```python
from build123d import *

# Parameters (mm, degrees)
SKETCH1_W           = 151.13
SKETCH1_H           = 82.55
BOSS_EXTRUDE1_DEPTH = 15.875
SKETCH2_W           = 167.005
SKETCH2_H           = 98.425
BOSS_EXTRUDE2_DEPTH = 3.81
FILLET2_R           = 6.35
CUT_EXTRUDE1_DEPTH  = 184.691243225
CUT_EXTRUDE3_DEPTH  = 5.4356
SKETCH5_W           = 8.89
SKETCH5_H           = 6.35
CUT_EXTRUDE4_DEPTH  = 189.417815482


with BuildPart() as part:
    # Sketch1 → Boss-Extrude1 (new body)
    with BuildSketch(Plane(origin=(0, 0, 0), x_dir=(1, 0, 0), z_dir=(0, 1, 0))):
        Polygon((-7.9375, 82.55), (-7.9375, -7.9375), (159.0675, -7.9375), (159.0675, 90.4875), (-7.9375, 90.4875), align=None)
        with Locations((75.565, 41.275)):
            Rectangle(SKETCH1_W, SKETCH1_H, mode=Mode.SUBTRACT)
    extrude(amount=BOSS_EXTRUDE1_DEPTH)

    # Sketch2 → Boss-Extrude2 (add)
    with BuildSketch(Plane.XZ):
        with Locations((75.565, -41.275)):
            Rectangle(SKETCH2_W, SKETCH2_H)
    extrude(amount=BOSS_EXTRUDE2_DEPTH)

    # Fillet2
    fillet2_edges = [part.edges().sort_by_distance(p)[0] for p in [
        (-7.9375, 6.0325, 7.9375),
        (-7.9375, 6.0325, -90.4875),
        (159.0675, 6.0325, -90.4875),
        (159.0675, 6.0325, 7.9375),
    ]]
    fillet(fillet2_edges, radius=FILLET2_R)

    # Sketch3 → Cut-Extrude1 (cut, through all)
    with BuildSketch(Plane.ZY.offset(-151.13)):
        with BuildLine():
            ThreePointArc((-58.8137, 7.9375), (-61.9125, 11.0363), (-65.0113, 7.9375))
            Line((-65.0113, 7.9375), (-58.8137, 7.9375))
        make_face()
        with BuildLine():
            Line((-58.8137, 7.9375), (-65.0113, 7.9375))
            ThreePointArc((-65.0113, 7.9375), (-61.9125, 4.8387), (-58.8137, 7.9375))
        make_face()
        with BuildLine():
            Line((-41.275, 7.9375), (-41.275, 11.0363))
            ThreePointArc((-41.275, 11.0363), (-43.466182494, 10.128682494), (-44.3738, 7.9375))
            Line((-44.3738, 7.9375), (-41.275, 7.9375))
        make_face()
        with BuildLine():
            Line((-41.275, 4.8387), (-41.275, 7.9375))
            Line((-41.275, 7.9375), (-44.3738, 7.9375))
            ThreePointArc((-44.3738, 7.9375), (-43.466182494, 5.746317506), (-41.275, 4.8387))
        make_face()
        with BuildLine():
            ThreePointArc((-38.1762, 7.9375), (-39.083817506, 10.128682494), (-41.275, 11.0363))
            Line((-41.275, 11.0363), (-41.275, 7.9375))
            Line((-41.275, 7.9375), (-38.1762, 7.9375))
        make_face()
        with BuildLine():
            Line((-38.1762, 7.9375), (-41.275, 7.9375))
            Line((-41.275, 7.9375), (-41.275, 4.8387))
            ThreePointArc((-41.275, 4.8387), (-39.083817506, 5.746317506), (-38.1762, 7.9375))
        make_face()
        with BuildLine():
            ThreePointArc((-23.7363, 7.9375), (-20.6375, 4.8387), (-17.5387, 7.9375))
            Line((-17.5387, 7.9375), (-23.7363, 7.9375))
        make_face()
        with BuildLine():
            Line((-23.7363, 7.9375), (-17.5387, 7.9375))
            ThreePointArc((-17.5387, 7.9375), (-20.6375, 11.0363), (-23.7363, 7.9375))
        make_face()
    extrude(amount=-CUT_EXTRUDE1_DEPTH, mode=Mode.SUBTRACT)

    # Sketch4 → Cut-Extrude3 (cut)
    with BuildSketch(Plane(origin=(0, 0, 0), x_dir=(0, 0, -1), z_dir=(1, 0, 0))):
        with BuildLine():
            Line((57.912502484, 13.869404287), (65.912502516, 13.869404287))
            ThreePointArc((65.912502516, 13.869404287), (67.326716079, 13.28361785), (67.912502516, 11.869404287))
            Line((67.912502516, 11.869404287), (70.412502516, 11.869404287))
            ThreePointArc((70.412502516, 11.869404287), (74.412502516, 7.869404287), (70.412502516, 3.869404287))
            Line((70.412502516, 3.869404287), (67.912502516, 3.869404287))
            ThreePointArc((67.912502516, 3.869404287), (67.326716079, 2.455190725), (65.912502516, 1.869404287))
            Line((65.912502516, 1.869404287), (57.912502484, 1.869404287))
            ThreePointArc((57.912502484, 1.869404287), (56.498288921, 2.455190725), (55.912502484, 3.869404287))
            Line((55.912502484, 3.869404287), (53.412502484, 3.869404287))
            ThreePointArc((53.412502484, 3.869404287), (49.412502484, 7.869404287), (53.412502484, 11.869404287))
            Line((53.412502484, 11.869404287), (55.912502484, 11.869404287))
            ThreePointArc((55.912502484, 11.869404287), (56.498288921, 13.28361785), (57.912502484, 13.869404287))
        make_face()
    extrude(amount=-CUT_EXTRUDE3_DEPTH, mode=Mode.SUBTRACT)

    # Sketch5 → Cut-Extrude4 (cut, through all)
    with BuildSketch(Plane(origin=(-5.4356, 0, 0), x_dir=(0, 0, -1), z_dir=(1, 0, 0))):
        with Locations((61.9125025, 7.869404287)):
            Rectangle(SKETCH5_W, SKETCH5_H)
    extrude(amount=-CUT_EXTRUDE4_DEPTH, mode=Mode.SUBTRACT)


solid = part.part
```
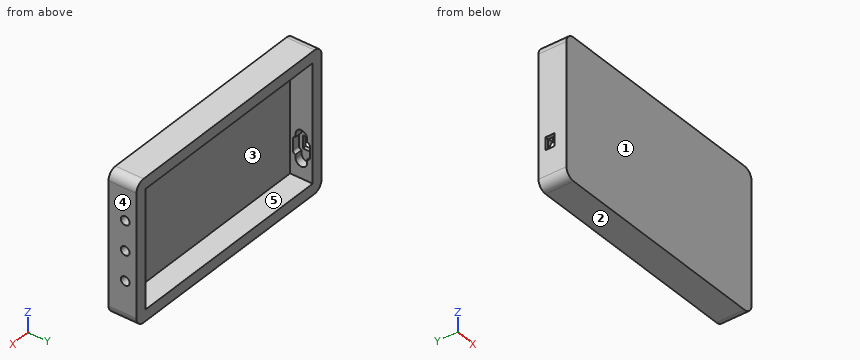
The listing builds one solid part. Answer for the finished solid, in the listing's coordinates (mm). Face numbers are marked on the shaded views. A direction names the side the tool comes from. Coordinates: 2 decimals unless noted, no trailing zeros. Write each loop counter-clockwise with the first axis right and the second up, starting at its lowest first coordinate (ties: lowest second). Pieces come first, ordered by that corner, then holes.
Q1. Find the intervals of material crossed by line 1 along Z through (x, y) = (120.5, 1.75); line 2 along X through (y, z) = (7.75, -27); line 3 along X through (y, z) = (12.75, -63), in increasing order.
Returned:
line 1: z = -90.49 to -82.55, 0 to 7.94
line 2: x = -7.94 to 0, 151.13 to 159.07
line 3: x = -7.94 to -5.44, 151.13 to 159.07
Q2. Section A-A, the plane z = -21.5 is taken. Write down the section's boundary in (x, y) (1 decimal), then the cut area to 3 significant figures.
Returned:
outline: (-7.9, -3.8) - (159.1, -3.8) - (159.1, 5) - (151.1, 5) - (151.1, 0) - (0, 0) - (0, 15.9) - (-7.9, 15.9) - close; (151.1, 10.9) - (159.1, 10.9) - (159.1, 15.9) - (151.1, 15.9) - close
area: 841 mm2
Q3. Which of the six approach directions +Z, -Z, +X, -X, +Y, -Y give full straight-line access (tool end or side, diameter ignored) to the marked faces 4 and 5?
Returned:
face 4: +Z, -Z, +X, +Y, -Y
face 5: +Y
Q4. The mould has two halves that part along Z. Classify the marked faces 1, 2 and 3: released by +Z, released by -Z, zero draft, split by the parting line, or undercut.
Returned:
face 1: zero draft
face 2: released by -Z
face 3: undercut
Q5. Given P1, Ø12, axis at x = 80, z = -25, coming from the +Y side; P2, Ø2, axis at x = -7, y = 9, coming from the +Z side, each flat-ended and moving along its own axis, determine where each tip first touches the part or whether it passes through.
Returned:
P1: stops at y = 0
P2: stops at z = 6.15
Q6. Section B-B, the plane z = -4 is taken. Write down the section's boundary in (x, y) (1 decimal).
Returned:
outline: (-7.9, -3.8) - (159.1, -3.8) - (159.1, 15.9) - (151.1, 15.9) - (151.1, 0) - (0, 0) - (0, 15.9) - (-7.9, 15.9) - close
